```python
from build123d import *

# Parameters (mm, degrees)
SKETCH1_R               = 12.25
BOSS_EXTRUDE1_DEPTH     = 380
CUT_EXTRUDE1_DEPTH      = 381.394696335
CUT_EXTRUDE1_DEPTH_BACK = 381.394696335
SKETCH2_R               = 2.5
CUT_EXTRUDE2_DEPTH      = 381.394696442
CUT_EXTRUDE2_DEPTH_BACK = 381.394696442
SKETCH3_R               = 10
CUT_EXTRUDE3_START      = -12.2500001
CUT_EXTRUDE3_OUTLINE_R  = 4
CUT_EXTRUDE3_DEPTH      = 3.08483721


# Read off the part's stored shape, not the designer's step: Cut-Extrude3
with BuildPart() as part:
    # Sketch1 → Boss-Extrude1 (new body)
    with BuildSketch(Plane.XY):
        Circle(SKETCH1_R)
    extrude(amount=BOSS_EXTRUDE1_DEPTH)

    # Sketch2 → Cut-Extrude1 (cut, two sides: drawn at the far end of the back side and taken through both)
    with BuildSketch(Plane(origin=(0, 0, 0), x_dir=(0, 0, -1), z_dir=(1, 0, 0)).offset(-CUT_EXTRUDE1_DEPTH_BACK)):
        with Locations((-370, 0)):
            Circle(SKETCH2_R)
    extrude(amount=CUT_EXTRUDE1_DEPTH + CUT_EXTRUDE1_DEPTH_BACK, mode=Mode.SUBTRACT)

    # Sketch3 → Cut-Extrude2 (cut, two sides: drawn at the far end of the back side and taken through both)
    with BuildSketch(Plane.XY.offset(380).offset(-CUT_EXTRUDE2_DEPTH_BACK)):
        Circle(SKETCH3_R)
    extrude(amount=CUT_EXTRUDE2_DEPTH + CUT_EXTRUDE2_DEPTH_BACK, mode=Mode.SUBTRACT)

    # Cut-Extrude3 outline → Cut-Extrude3 (cut)
    with BuildSketch(Plane(origin=(0, 0, 0), x_dir=(1, 0, 0), z_dir=(0, 1, 0)).offset(CUT_EXTRUDE3_START)):
        with Locations((0, -20)):
            Circle(CUT_EXTRUDE3_OUTLINE_R)
    extrude(amount=CUT_EXTRUDE3_DEPTH, mode=Mode.SUBTRACT)


solid = part.part
```
For this review, take the finished solid that the model builds, in its own axes (mm). Give positions to 0.01 mm unless a question says otherwise; leave off trailing zeros. Loops run counter-clockwise (first coordinate to the right, second up) from the corner with the lowest first, then second, coordinate; pieces in that order, holes last. Notation, with made-up numbers: M 47.5,-22 L 102.5,-22 A18 cw 102.5,-16 Z; hole C 2.25,61 d1. An arc over 180 degrees is marked long. One line per item, written item: value. Start each with the question number.
Q1. Add section B-B (z = 104). Give the boundary of the cut face in (x, y), and give its area (3 significant figures).
Q2. Clearance check with flat-ended pins moving along their axes: pin 1 Ø4.5 at (y, z) = (0, 370) entering from +X; pin 2 Ø5 at (x, z) = (-3, 55.5) entering from +Y; pin 3 Ø8 at (x, z) = (9, 299.5) entering from -Y; pin 4 Ø6 at (y, z) = (-5, 125) entering from -X. State where each tip first meets the part, or that it passes through.
Q3. Add section A-A (x = 0). Give the boundary of the cut face in (y, z).
Q4. For L1, parallel to Y at x = 0, z = 129.5; L2, parallel to X at y = 0.5, z = 325.5; L3, parallel to Z at x = 10.9, y = 0, list the stretches that pass through material, from the lowest coordinate up.
Q5. Draft analysis for pull direction Z (two halves, no side actions). For faces 1 (the face through (-5, -9, 0)), 2 (the face through (-3.2, -10.7, 22.4)), 3 (the face through (-5, -9, 380)), state which applies: released by +Z, released by -Z, zero draft, split by the parting line, or undercut.
Reply:
1. outline: C 0,0 d24.5; hole C 0,0 d20
1. area: 157 mm²
2. pin 1: through
2. pin 2: y = 12.24
2. pin 3: y = -11.18
2. pin 4: x = -12.09
3. outline: M -12.25,0 L -10,0 L -10,16 L -12.25,16 Z; M -12.25,24 L -10,24 L -10,380 L -12.25,380 Z; M 10,0 L 12.25,0 L 12.25,380 L 10,380 Z
4. L1: -12.25 to -10, 10 to 12.25
4. L2: -12.24 to -9.99, 9.99 to 12.24
4. L3: 0 to 367.5, 372.5 to 380
5. face 1: released by -Z
5. face 2: undercut
5. face 3: released by +Z
